```python
from build123d import *

# Parameters (mm, degrees)
SKETCH014_W     = 210
SKETCH014_H     = 70
PAD004_DEPTH    = 8
SKETCH015_W     = 210
SKETCH015_H     = 70
SKETCH015_W_2   = 189.4
SKETCH015_H_2   = 49.4
POCKET006_DEPTH = 3
SKETCH016_R     = 1.3
POCKET007_DEPTH = 25


with BuildPart() as part:
    # Sketch014 → Pad004 (new body)
    with BuildSketch(Plane.XY):
        with Locations((105, -35)):
            Rectangle(SKETCH014_W, SKETCH014_H)
    extrude(amount=PAD004_DEPTH)

    # Sketch015 (on Face6 of Pad004) → Pocket006 (cut)
    with BuildSketch(Plane.XY.offset(8)):
        with Locations((105, -35)):
            Rectangle(SKETCH015_W, SKETCH015_H)
        with Locations((105, -35)):
            Rectangle(SKETCH015_W_2, SKETCH015_H_2, mode=Mode.SUBTRACT)
    extrude(amount=-POCKET006_DEPTH, mode=Mode.SUBTRACT)

    # Sketch016 (on Face11 of Pocket006) → Pocket007 (cut)
    with BuildSketch(Plane.XY.offset(8)):
        with Locations((5, -5)):
            Circle(SKETCH016_R)
        with Locations((205, -5)):
            Circle(SKETCH016_R)
        with Locations((205, -65)):
            Circle(SKETCH016_R)
        with Locations((5, -65)):
            Circle(SKETCH016_R)
    extrude(amount=-POCKET007_DEPTH, mode=Mode.SUBTRACT)


solid = part.part
```
Part model, mm, in its own coordinate system. Round coordinates to 2 decimals unless told otherwise and drop trailing zeros. Order: outer loops, then holes, each group sorted by start corner. A loop starts at its lowest first (then second) coordinate and runs counter-clockwise, first axis right, second up. Notation, with made-up numbers: M -34,14 L -6,14 A16 ccw -6,44 Z; hole C -4.5,-36.75 d4. An arc over 180 degrees is marked long. Answer in a Markdown table with one row per item. Add a question column.
Q1. Cut at A-A on y = -35.5. Give the cut face in (x, z).
Q2. Wall check: L1, parallel to Y at x = 205, z = 3; L2, parallel to X at y = -65, z = 4; L3, parallel to X at y = -4, z = 1.25. Give the ranges that are in metal, low to high. Write a range as from..to.
Q3. Pin check, flat tips, straight feed: pin 1 (2.5 mm diameter, centred on x = 135, z = 7, fed in from +Y); pin 2 (4 mm diameter, centred on x = 5, y = -65, fed in from -Z); pin 3 (0.9 mm diameter, centred on y = -28, z = 7, fed in from -X); pin 4 (0.9 mm diameter, centred on x = 68, z = 6.5, fed in from -Y). Stop position of each tip, or through.
Q4. Cut at B-B on x = 14. Give the cut face in (y, z).
Established:
| question | item | result |
|---|---|---|
| 1 | outline | M 0,0 L 210,0 L 210,5 L 199.7,5 L 199.7,8 L 10.3,8 L 10.3,5 L 0,5 Z |
| 2 | L1 | y = -70..-66.3, -63.7..-6.3, -3.7..0 |
| 2 | L2 | x = 0..3.7, 6.3..203.7, 206.3..210 |
| 2 | L3 | x = 0..4.17, 5.83..204.17, 205.83..210 |
| 3 | pin 1 | stops at y = -10.3 |
| 3 | pin 2 | stops at z = 0 |
| 3 | pin 3 | stops at x = 10.3 |
| 3 | pin 4 | stops at y = -59.7 |
| 4 | outline | M -70,0 L 0,0 L 0,5 L -10.3,5 L -10.3,8 L -59.7,8 L -59.7,5 L -70,5 Z |
